from build123d import *

# Parameters (mm, degrees)
PADR_OCIRCULAR1_COUNT = 4
FILETE1_R             = 0.5


with BuildPart() as part:
    # Esboço1 → Revolução1 (revolve)
    with BuildSketch(Plane(origin=(0, 0, 0), x_dir=(0, 0, -1), z_dir=(1, 0, 0)), mode=Mode.PRIVATE) as revolu_o1_sk:
        Polygon((0, 10), (0, 12.75), (-0.5, 12.75), (-0.5, 13.25), (0, 13.25), (0, 15.5), (-0.5, 15.5), (-0.5, 16), (0, 16), (0, 27), (-8, 27), (-8, 16), (-42, 16), (-42, 13.25), (-41.5, 13.25), (-41.5, 12.75), (-42, 12.75), (-42, 10), align=None)
    revolve(revolu_o1_sk.sketch.rotate(Axis((0, 0, 0), (0, 0, 1)), 90), axis=Axis((0, 0, 0), (0, 0, 1)))  # turned: the seam where the file's is

    # Esboço5 → Corte-Revolução1 (revolve, cut)
    with BuildSketch(Plane(origin=(0, 0, 0), x_dir=(0, 0, -1), z_dir=(1, 0, 0)), mode=Mode.PRIVATE) as corte_revolu_o1_sk:
        Polygon((0, 26), (-5.1, 26), (-5.1, 24.25), (-8, 24.25), (-8, 21.5), (0, 21.5), align=None)
    corte_revolu_o1 = revolve(corte_revolu_o1_sk.sketch.rotate(Axis((0, 21.5, 0), (0, 0, -1)), 90), axis=Axis((0, 21.5, 0), (0, 0, -1)), mode=Mode.SUBTRACT)  # turned: the seam where the file's is

    # PadrãoCircular1: Corte-Revolução1 ×4 about axis
    padr_ocircular1_axis = Axis((0, 0, 0), (0, 0, 1))
    for i in range(1, PADR_OCIRCULAR1_COUNT):
        add(corte_revolu_o1.rotate(padr_ocircular1_axis, i * 360 / PADR_OCIRCULAR1_COUNT), mode=Mode.SUBTRACT)

    # Filete1
    filete1_edges = [part.edges().sort_by_distance(p)[0] for p in [
        (16, 0, 42),
        (27, 0, 8),
        (27, 0, 0),
    ]]
    fillet(filete1_edges, radius=FILETE1_R)


solid = part.part
Could you check a few things on this model? Use its own coordinates, in mm. A direction names the side the tool comes from. Give positions to 0.01 mm unless a question says otherwise; leave off trailing zeros. Loops run counter-clockwise (first coordinate to the right, second up) from the corner with the lowest first, then second, coordinate; pieces in that order, holes last. Notation, with made-up numbers: (25.25, 15.5) -> (63.25, 15.5) arc R29 cw to (63.25, 42.5) -> close; hole circle Ø4 at (-29.5, 50). An arc over 180 degrees is marked (long way). Answer as CSV lines item,"result". Start each with the question number.
(1) If we section it at C-C on z = 31: Write out the boundary of the cut face in (x, y), then the cut area to 3 significant figures.
(2) I need wall thicknesses on probe 1 along Y at (x, z) = (0, 3); probe 2 along Y at (x, z) = (0, 6); probe 3 along Y at (x, z) = (-21, 6). Which ranges of each line are inside material? Lowest first, please.
(3) If we section it at A-A on z = 4: Write out the boundary of the cut face in (x, y), then the cut area to 3 significant figures.
(4) I'm going to push flat-ended pins straight in: pin 1 Ø5 at (x, y) = (0, 21.5) entering from -Z; pin 2 Ø1 at (x, y) = (18.5, -7.5) entering from +Z; pin 3 Ø12 at (x, z) = (-6, 6) entering from -Y; pin 4 Ø12 at (x, z) = (14.5, 29.5) entering from +Y. Where does each tip first touch, or does it pass through?
(5) We'd pull the mould along Y, two halves only. Please class faces 4 (the cylindrical face through (5.85, 26.36, 4.05)), 5 (the cylindrical face through (-2.419, -17.706, 2.586)), 6 (the flat face through (-12, 11, 0)): released by +Y, released by -Y, zero draft, split by the parting line, or undercut.
(6) If we section it at B-B on y = 0: Count the separate pieces of the cut face and the enclosed holes in it, then the cut area to 3 significant figures.
(7) Which directions (+Z, -Z, +X, -X, +Y, -Y) give clear straight access to the entire face, cutting with the end or side of a thin tool? Please do faces 1 (the flat face through (13, -5, 0)), 2 (the flat face through (-19, 2, 5.1)), 3 (the cylindrical face through (1.725, -13.137, 41.746)).
Computed:
1,outline,"circle Ø32 at (0, 0); hole circle Ø20 at (0, 0)"
1,area,"490 mm2"
2,probe 1,"y = -27 to -26, -17 to -10, 10 to 17, 26 to 27"
2,probe 2,"y = -27 to -24.25, -18.75 to -10, 10 to 18.75, 24.25 to 27"
2,probe 3,"y = -16.97 to -2.7, 2.7 to 16.97"
3,outline,"circle Ø54 at (0, 0); hole circle Ø9 at (-21.5, 0); hole circle Ø20 at (0, 0); hole circle Ø9 at (0, -21.5); hole circle Ø9 at (0, 21.5); hole circle Ø9 at (21.5, 0)"
3,area,"1,720 mm2"
4,pin 1,"passes through"
4,pin 2,"stops at z = 8"
4,pin 3,"stops at y = -27"
4,pin 4,"stops at y = 13.56"
5,face 4,"split by the parting line"
5,face 5,"undercut"
5,face 6,"zero draft"
6,separate pieces,"4"
6,enclosed holes,"0"
6,area,"554 mm2"
7,face 1,"-Z, +X, -X, +Y, -Y"
7,face 2,"-Z"
7,face 3,"+Z"
